Here's how the part is built. I have some questions about the finished solid (model axes, mm). A direction names the side the tool comes from. Coordinates: 2 decimals unless noted, no trailing zeros. Write each loop counter-clockwise with the first axis right and the second up, starting at its lowest first coordinate (ties: lowest second). Pieces come first, ordered by that corner, then holes.
(1) Imagine slicing it at C-C, the plane z = 0.95. List the corners of the cut face in (x, y) for me.
(2) Thinking about a two-plate mould opening in X: for faces 4 (the flat face through (-4, -50, 2)), 5 (the flat face through (-9, -51, 2)), 6 (the cylindrical face through (-9.38, -47.71, 1.67)), which applies, released by +X, released by -X, zero draft, split by the parting line, or undercut?
(3) Please list where these lines run through material, in increasing order: probe 1 along Y at (x, z) = (-9, 2.45); probe 2 along Y at (x, z) = (9, 1); probe 3 along Y at (x, z) = (-0.5, 2.8).
(4) Imagine slicing it at A-A, the plane y = 26. List the corners of the cut face in (x, z) for me.
(5) Which directions (+Z, -Z, +X, -X, +Y, -Y) give clear straight access to the entire face, cutting with the end or side of a thin tool? Please do faces 1 (the cylindrical face through (8.62, 44.29, 1.67)), 2 (the flat face through (3, 46, 2)), 3 (the flat face through (-3, -47, 2)).
(6) For pin 1 Ø1 at (y, z) = (-47.5, 1) entering from +X; pin 2 Ø1.6 at (x, z) = (-7.5, 1) entering from +Y; pin 3 Ø1.6 at (y, z) = (47.5, 1) entering from -X, each with a flat end and sliding along its axis, tell me the tip position at first contact or that it passes through.
(7) Imagine slicing it at B-B, the plane x = 9. List the corners of the cut face in (y, z) for me.
```python
from build123d import *

# Parameters (mm, degrees)
F0_W      = 12
F0_H      = 10
F1_DEPTH  = 3.3
F2_SIZE   = 2
F3_R      = 3
F4_R      = 3
F5_R      = 1.75
F6_DEPTH  = 25
F7_R      = 2.5
F8_DEPTH  = 25
F9_R      = 4.25
F10_DEPTH = 25


with BuildPart() as f1:
    # F0 (on Top) → F1 (new body)
    with BuildSketch(Plane.XY):
        Polygon((15, -41), (15, 41), (3, 41), (-15, 41), (-15, -41), (-3, -41), align=None)
        with Locations((9, 46)):
            Rectangle(F0_W, F0_H)
        with Locations((-9, -46)):
            Rectangle(F0_W, F0_H)
    extrude(amount=F1_DEPTH)

    # F2
    f2_edges = [f1.edges().sort_by_distance(p)[0] for p in [
        (15, 51, 1.65),
        (3, 51, 1.65),
        (-15, -51, 1.65),
        (-3, -51, 1.65),
    ]]
    chamfer(f2_edges, length=F2_SIZE)

    # F3
    f3_edges = [f1.edges().sort_by_distance(p)[0] for p in [
        (3, 41, 1.65),
    ]]
    fillet(f3_edges, radius=F3_R)

    # F4
    f4_edges = [f1.edges().sort_by_distance(p)[0] for p in [
        (-3, -41, 1.65),
    ]]
    fillet(f4_edges, radius=F4_R)

    # F5 (on face) → F6 (cut)
    with BuildSketch(Plane.XY.offset(3.3)):
        with Locations((9, 46)):
            Circle(F5_R)
        with Locations((-9, -46)):
            Circle(F5_R)
    extrude(amount=-F6_DEPTH, mode=Mode.SUBTRACT)

    # F7 (on face) → F8 (cut)
    with BuildSketch(Plane.XY.offset(3.3)):
        with Locations((0, 26)):
            Circle(F7_R)
        with Locations((0, -26)):
            Circle(F7_R)
    extrude(amount=-F8_DEPTH, mode=Mode.SUBTRACT)

    # F9 (on face) → F10 (cut)
    with BuildSketch(Plane.XY.offset(3.3)):
        with Locations((0, 26)):
            Circle(F9_R)
        with Locations((0, -26)):
            Circle(F9_R)
    extrude(amount=-F10_DEPTH, mode=Mode.SUBTRACT)


solid = f1.part
```
Recorded:
1. outline: (-15, -49) - (-13, -51) - (-5, -51) - (-3, -49) - (-3, -44) arc R3 cw to (0, -41) - (15, -41) - (15, 49) - (13, 51) - (5, 51) - (3, 49) - (3, 44) arc R3 cw to (0, 41) - (-15, 41) - close; hole circle Ø3.5 at (-9, -46); hole circle Ø8.5 at (0, -26); hole circle Ø8.5 at (0, 26); hole circle Ø3.5 at (9, 46)
2. face 4: released by +X
2. face 5: zero draft
2. face 6: undercut
3. probe 1: y = -51 to -47.75, -44.25 to 41
3. probe 2: y = -41 to 44.25, 47.75 to 51
3. probe 3: y = -41.04 to -30.22, -21.78 to 21.78, 30.22 to 41
4. outline: (-15, 0) - (-4.25, 0) - (-4.25, 3.3) - (-15, 3.3) - close; (4.25, 0) - (15, 0) - (15, 3.3) - (4.25, 3.3) - close
5. face 1: +Z, -Z
5. face 2: +Z, -Z, -X, +Y
5. face 3: +Z, -Z, +X, -Y
6. pin 1: stops at x = -3
6. pin 2: stops at y = 41
6. pin 3: stops at x = 3
7. outline: (-41, 0) - (44.25, 0) - (44.25, 3.3) - (-41, 3.3) - close; (47.75, 0) - (51, 0) - (51, 3.3) - (47.75, 3.3) - close
